Could you check a few things on this model? Use its own coordinates, in mm. Face numbers are marked on the shaded views. A direction names the side the tool comes from. Give positions to 0.01 mm unless a question says otherwise; leave off trailing zeros. Loops run counter-clockwise (first coordinate to the right, second up) from the corner with the lowest first, then second, coordinate; pieces in that order, holes last. Notation, with made-up numbers: M 45,-37.5 L 95,-37.5 A17 cw 95,-23.5 Z; hole C 79,12.25 d4. An arc over 180 degrees is marked long. Return JSON: item names as keys, results as strings. Group by question number.
1. For the marked faces 1, 2, 3 and 4, which set-ups out of +Z, -Z, +X, -X, +Y, -Y let a thin tool reach every point of the face, with its end or its side?
2. Please list where these lines run through material, in increasing order: line 1 (Z direction, x = 3.75, y = 4); line 2 (X direction, y = 11.7, z = -1); line 3 (Z direction, x = 1, y = 2).
3. If we section it at B-B (z = -6.25): Write out the boundary of the cut face in (x, y).
4. If we section it at C-C (x = 3.2): Write out the boundary of the cut face in (y, z).
5. For pin 1 (2.5 mm diameter, centred on x = 4, y = 11, fed in from +Z); pin 2 (1 mm diameter, centred on x = 3.5, y = 9, fed in from +Z); pin 3 (1.1 mm diameter, centred on x = 4.5, z = -6.5, fed in from +Y), each with a flat end and sliding along its axis, tell me the tip position at first contact or that it passes through.
6. If we mould it in two halves opening along Z, with no side actions, what happens to the marked faces 5, 6, 7 and 8? For each: +Z half, -Z half, draft (parallel to the pull), parting line (faces both ways), or undercut.
7. If we section it at D-D (z = -1.75): Write out the boundary of the cut face in (x, y), plus the area to 3 significant figures.
8. If we section it at A-A (y = 4.75): Write out the boundary of the cut face in (x, z), plus the area to 3 significant figures.
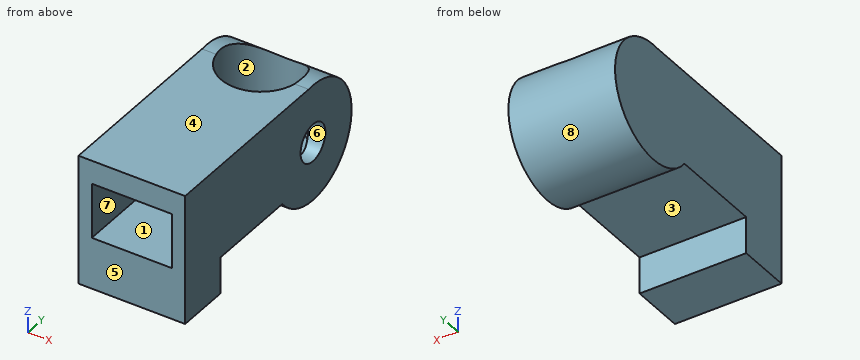
```python
from build123d import *

# Parameters (mm, degrees)
BOSS_EXTRUDE1_DEPTH = 6.4
SKETCH2_R           = 1.125
CUT_EXTRUDE1_DEPTH  = 2
SKETCH4_R           = 2.4
CUT_EXTRUDE3_DEPTH  = 5
SKETCH5_W           = 4.8
SKETCH5_H           = 3.3
CUT_EXTRUDE4_DEPTH  = 8.9


with BuildPart() as part:
    # Sketch1 → Boss-Extrude1 (new body)
    with BuildSketch(Plane(origin=(0, 0, 0), x_dir=(0, 0, -1), z_dir=(1, 0, 0))):
        with BuildLine():
            Line((0, 0), (7.8, 0))
            Line((7.8, 0), (7.8, 3.2))
            Line((7.8, 3.2), (5.6, 3.2))
            Line((5.6, 3.2), (5.6, 8.8))
            ThreePointArc((5.6, 8.8), (4.857585772, 14.801033467), (0, 11.2))
            Line((0, 11.2), (0, 0))
        make_face()
    extrude(amount=BOSS_EXTRUDE1_DEPTH)

    # Sketch2 → Cut-Extrude1 (cut)
    with BuildSketch(Plane(origin=(6.4, 0, 0), x_dir=(0, 0, -1), z_dir=(1, 0, 0))):
        with Locations((3.478868227, 11.584025862)):
            Circle(SKETCH2_R)
    extrude(amount=-CUT_EXTRUDE1_DEPTH, mode=Mode.SUBTRACT)

    # Sketch4 → Cut-Extrude3 (cut, symmetric)
    with BuildSketch(Plane.XY):
        with Locations((3.2, 11.7)):
            Circle(SKETCH4_R)
    extrude(amount=CUT_EXTRUDE3_DEPTH, both=True, mode=Mode.SUBTRACT)

    # Sketch5 → Cut-Extrude4 (cut)
    with BuildSketch(Plane.XZ):
        with Locations((3.2, -3.05)):
            Rectangle(SKETCH5_W, SKETCH5_H)
    extrude(amount=-CUT_EXTRUDE4_DEPTH, mode=Mode.SUBTRACT)


solid = part.part
```
Answer:
{
 "1": {"face 1": "-Y", "face 2": "+Z", "face 3": "-Z, +X, -X", "face 4": "+Z, +X, -X, -Y"},
 "2": {"line 1": "z = -5.6 to -4.7, -1.4 to 0", "line 2": "x = 0 to 0.8, 5.6 to 6.4", "line 3": "z = -7.8 to -4.7, -1.4 to 0"},
 "3": {"outline": "M 0,0 L 6.4,0 L 6.4,3.2 L 0,3.2 Z; M 0,9.45 L 6.4,9.45 L 6.4,13.72 L 0,13.72 Z"},
 "4": {"outline": "M 0,-7.8 L 3.2,-7.8 L 3.2,-5.6 L 8.8,-5.6 A3.5 ccw long 14.1,-1.05 L 14.1,-5 L 9.3,-5 L 9.3,0 L 0,0 L 0,-1.4 L 8.9,-1.4 L 8.9,-4.7 L 0,-4.7 Z"},
 "5": {"pin 1": "stops at z = -5", "pin 2": "stops at z = 0", "pin 3": "stops at y = 14.06"},
 "6": {"face 5": "draft", "face 6": "undercut", "face 7": "undercut", "face 8": "parting line"},
 "7": {"outline": "M 0,0 L 0.8,0 L 0.8,8.9 L 5.6,8.9 L 5.6,0 L 6.4,0 L 6.4,14.63 L 0,14.63 Z; hole C 3.2,11.7 d4.8", "area": "32.8 mm²"},
 "8": {"outline": "M 0,-5.6 L 6.4,-5.6 L 6.4,0 L 0,0 Z; hole M 0.8,-4.7 L 5.6,-4.7 L 5.6,-1.4 L 0.8,-1.4 Z", "area": "20.0 mm²"}
}
